Check sheet for the drawn part. Datum: minimum x, y, z corner. Units: mm. A direction names the side the tool comes from. Coordinates: 2 decimals unless noted, no trailing zeros. Order: outer loops, then holes, each group sorted by start corner. A loop starts at its lowest first (then second) coordinate and runs counter-clockwise, first axis right, second up. Notation, with made-up numbers: (-39, -1.75) - (-19, -1.75) arc R18 cw to (-19, 25.25) - close; hole circle Ø10 at (-12, 42.5). An arc over 180 degrees is marked (long way). Return JSON: item names as keys, results as strings. Group by question number.
Item 1: Section check C-C on y = 62.5. Enter the section's corners in (x, z).
Item 2: Gauge pin test, flat ends, axial feed: pin 1 (3 mm diameter, centred on x = 10, y = 10, fed in from -Z); pin 2 (1.2 mm diameter, centred on y = 62, z = 1.5, fed in from +X). Record the tip position at first contact, or that the pin passes through.
Item 3: Scan lines: probe 1 along Y at (x, z) = (10, 2.55); probe 2 along Y at (x, z) = (40, 2.1); probe 3 along Y at (x, z) = (9, 1.8). Record each from-to range of solid material in increasing order.
Item 4: Section check A-A on x = 10. Enter the section's corners in (y, z).
Item 5: Section check B-B on z = 1.9. Enter the section's corners in (x, y).
Item 6: Section check D-D on x = 40. Enter the section's corners in (y, z).
Item 7: Tool access check on the marked faces 1 and 2. Record the directions out of +Z, -Z, +X, -X, +Y, -Y that give a thin tool (end or side, any length) a straight path to the whole face; none if there is none.
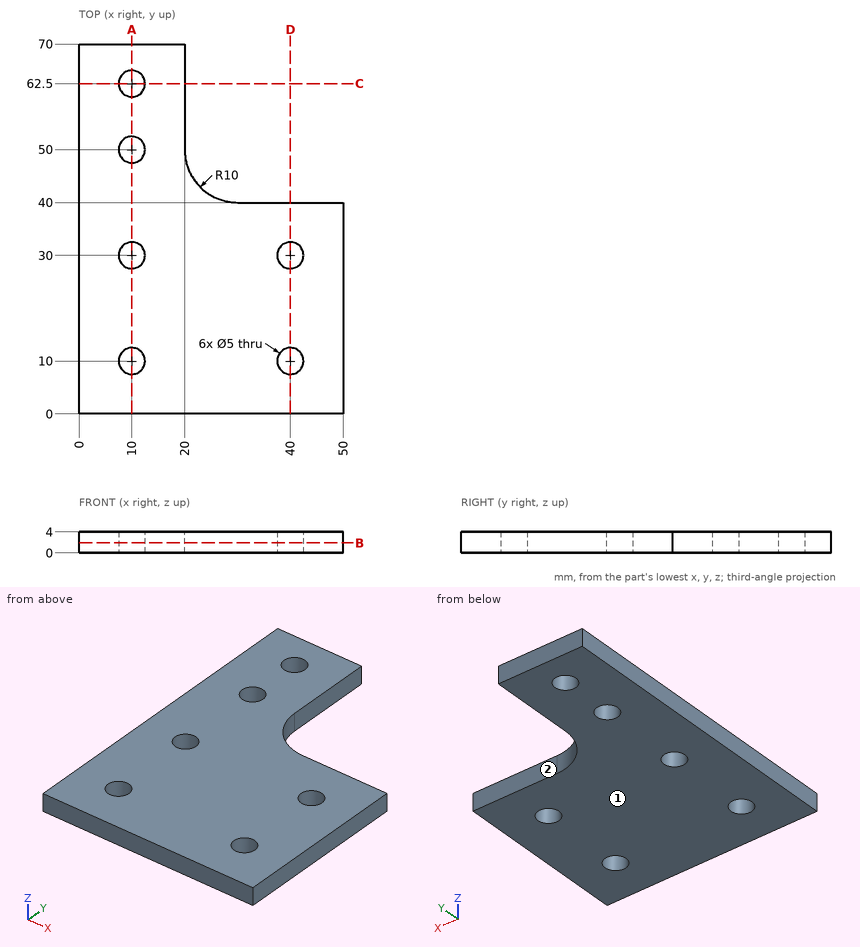
Computed:
{
 "1": {"outline": "(0, 0) - (7.5, 0) - (7.5, 4) - (0, 4) - close; (12.5, 0) - (20, 0) - (20, 4) - (12.5, 4) - close"},
 "2": {"pin 1": "passes through", "pin 2": "stops at x = 20"},
 "3": {"probe 1": "y = 0 to 7.5, 12.5 to 27.5, 32.5 to 47.5, 52.5 to 60, 65 to 70", "probe 2": "y = 0 to 7.5, 12.5 to 27.5, 32.5 to 40", "probe 3": "y = 0 to 7.71, 12.29 to 27.71, 32.29 to 47.71, 52.29 to 60.21, 64.79 to 70"},
 "4": {"outline": "(0, 0) - (7.5, 0) - (7.5, 4) - (0, 4) - close; (12.5, 0) - (27.5, 0) - (27.5, 4) - (12.5, 4) - close; (32.5, 0) - (47.5, 0) - (47.5, 4) - (32.5, 4) - close; (52.5, 0) - (60, 0) - (60, 4) - (52.5, 4) - close; (65, 0) - (70, 0) - (70, 4) - (65, 4) - close"},
 "5": {"outline": "(0, 0) - (50, 0) - (50, 40) - (30, 40) arc R10 cw to (20, 50) - (20, 70) - (0, 70) - close; hole circle Ø5 at (10, 10); hole circle Ø5 at (10, 30); hole circle Ø5 at (10, 50); hole circle Ø5 at (10, 62.5); hole circle Ø5 at (40, 10); hole circle Ø5 at (40, 30)"},
 "6": {"outline": "(0, 0) - (7.5, 0) - (7.5, 4) - (0, 4) - close; (12.5, 0) - (27.5, 0) - (27.5, 4) - (12.5, 4) - close; (32.5, 0) - (40, 0) - (40, 4) - (32.5, 4) - close"},
 "7": {"face 1": "-Z, +X, -X, +Y, -Y", "face 2": "+Z, -Z, +X, +Y"}
}
